For this review, take the finished solid that the model builds, in its own axes (mm). A direction names the side the tool comes from. Round coordinates to 2 decimals unless told otherwise and drop trailing zeros. Loops run counter-clockwise (first coordinate to the right, second up) from the corner with the lowest first, then second, coordinate; pieces in that order, holes last.
```python
from build123d import *
from OCP.BRepFilletAPI import BRepFilletAPI_MakeChamfer

# Parameters (mm, degrees)
ESQUISSE2_W             = 25
ESQUISSE2_H             = 36
BOSS_EXTRU_1_DEPTH      = 1.5
ESQUISSE3_W             = 3.350614404
ESQUISSE3_H             = 24
ESQUISSE3_W_2           = 3.329385596
BOSS_EXTRU_2_DEPTH      = 1.5
BOSS_EXTRU_3_DEPTH      = 8.58
BOSS_EXTRU_3_DEPTH_BACK = 3
BOSS_EXTRU_4_START      = 2.5
ESQUISSE5_W             = 18.32
ESQUISSE5_H             = 3
BOSS_EXTRU_4_DEPTH      = 6.08
ESQUISSE6_W             = 16.5
ESQUISSE6_H             = 1.5
BOSS_EXTRU_5_DEPTH      = 8
ESQUISSE7_W             = 25
ESQUISSE7_H             = 18
ENL_V_MAT_EXTRU_1_DEPTH = 5
CHANFREIN1_SIZE         = 10
CHANFREIN1_SIZE_2       = 5
CHANFREIN3_SIZE         = 3
CONG_1_R                = 3
CONG_2_R                = 3
D_GAGEMENT_M31_D        = 3.4


# Some blends are built 0.0001 mm under size
with BuildPart() as part:
    # Esquisse2 → Boss.-Extru.1 (new body)
    with BuildSketch(Plane.XY):
        with Locations((0, -137)):
            Rectangle(ESQUISSE2_W, ESQUISSE2_H)
    extrude(amount=BOSS_EXTRU_1_DEPTH)

    # Esquisse3 → Boss.-Extru.2 (add)
    with BuildSketch(Plane.XY.offset(1.5)):
        with Locations((10.824692798, -131)):
            Rectangle(ESQUISSE3_W, ESQUISSE3_H)
        Polygon((-12.5, -143), (-12.5, -155), (12.5, -155), (12.5, -143), (9.149385596, -143), (-9.170614404, -143), align=None)
        with Locations((-10.835307202, -131)):
            Rectangle(ESQUISSE3_W_2, ESQUISSE3_H)
    extrude(amount=BOSS_EXTRU_2_DEPTH)

    # Esquisse4 → Boss.-Extru.3 (add, two sides: drawn at the far end of the back side and taken through both)
    with BuildSketch(Plane.XY.offset(3).offset(-BOSS_EXTRU_3_DEPTH_BACK)):
        Polygon((-12.5, -119), (-15.5, -119), (-12.5, -137), (-12.5, -155), (12.5, -155), (12.5, -137), (15.5, -119), (12.5, -119), (10.747346399, -119), (10.747346399, -146), (-10.752653601, -146), (-10.752653601, -119), align=None)
    extrude(amount=BOSS_EXTRU_3_DEPTH + BOSS_EXTRU_3_DEPTH_BACK)

    # Esquisse5 → Boss.-Extru.4 (add)
    with BuildSketch(Plane.XY.offset(3).offset(BOSS_EXTRU_4_START)):
        Polygon((-10.752653601, -140), (-10.752653601, -146), (10.747346399, -146), (10.747346399, -140), (9.149385596, -140), (9.149385596, -143), (-9.170614404, -143), (-9.170614404, -140), align=None)
        with Locations((-0.010614404, -141.5)):
            Rectangle(ESQUISSE5_W, ESQUISSE5_H)
    extrude(amount=BOSS_EXTRU_4_DEPTH)

    # Esquisse6 → Boss.-Extru.5 (add)
    with BuildSketch(Plane(origin=(0, -119, 0), x_dir=(1, 0, 0), z_dir=(0, 1, 0))):
        Polygon((8.247346399, -11.58), (10.747346399, -11.58), (10.747346399, -5.5), (8.247346399, -5.5), (8.247346399, -10.08), align=None)
        with Locations((-0.002653601, -10.83)):
            Rectangle(ESQUISSE6_W, ESQUISSE6_H)
        Polygon((-10.752653601, -11.58), (-8.252653601, -11.58), (-8.252653601, -10.08), (-8.252653601, -5.5), (-10.752653601, -5.5), align=None)
    extrude(amount=-BOSS_EXTRU_5_DEPTH)

    # Esquisse7 → Enlèv. mat.-Extru.1 (cut)
    with BuildSketch(Plane.XY.offset(11.58)):
        with Locations((0, -146)):
            Rectangle(ESQUISSE7_W, ESQUISSE7_H)
    extrude(amount=-ENL_V_MAT_EXTRU_1_DEPTH, mode=Mode.SUBTRACT)

    # Chanfrein1
    chanfrein1_edges_1 = [part.edges().sort_by_distance(p)[0] for p in [
        (11.6236732, -137, 11.58),
    ]]
    chanfrein1_side_1 = [part.faces().sort_by_distance(p)[0] for p in [
        (11.6236732, -136.9, 11.58),
    ]]
    chanfrein1_edges_2 = [part.edges().sort_by_distance(p)[0] for p in [
        (-11.6263268, -137, 11.58),
    ]]
    chanfrein1_side_2 = [part.faces().sort_by_distance(p)[0] for p in [
        (-11.6263268, -136.9, 11.58),
    ]]
    chanfrein1 = BRepFilletAPI_MakeChamfer(part.part.solid().wrapped)
    for e in chanfrein1_edges_1:
        chanfrein1.Add(CHANFREIN1_SIZE - 0.0001, CHANFREIN1_SIZE_2 - 0.0001, e.wrapped, chanfrein1_side_1[0].wrapped)
    for e in chanfrein1_edges_2:
        chanfrein1.Add(CHANFREIN1_SIZE - 0.0001, CHANFREIN1_SIZE_2 - 0.0001, e.wrapped, chanfrein1_side_2[0].wrapped)
    add(Compound.cast(chanfrein1.Shape()), mode=Mode.REPLACE)  # a hair under: the kernel refuses the full size

    # Chanfrein3
    # the kernel refuses this chamfer: 3 mm, written as the material it adds along each edge
    with BuildSketch(Plane(origin=(-10.752653601, -127, 5.5), x_dir=(0.9996219169112968, 0.027495876610586775, 0), z_dir=(0, 0, 1))) as chanfrein3_piece_1_section:
        Polygon((CHANFREIN3_SIZE * 0.999621916911, -CHANFREIN3_SIZE * 0.0274958766106), (-CHANFREIN3_SIZE * 0.0274958766106, -CHANFREIN3_SIZE * 0.999621916911), (0, 0), align=None)
    chanfrein3_piece_1 = extrude(amount=6.08, mode=Mode.PRIVATE)
    chanfrein3_piece_1 = split(chanfrein3_piece_1, bisect_by=Plane(origin=(-8.784858651, -128.928894575, 10.615612357), z_dir=(0, 0.4472100177446834, -0.8944289798686087)), keep=Keep.TOP, mode=Mode.PRIVATE)
    chanfrein3_piece_1 = split(chanfrein3_piece_1, bisect_by=Plane(origin=(-8.252653601, -127.516102525, 7.79), z_dir=(-1, 0, 0)), keep=Keep.TOP, mode=Mode.PRIVATE)
    add(chanfrein3_piece_1)
    with BuildSketch(Plane(origin=(-10.752653601, -127, -2.215048964), x_dir=(0.9996219169112968, 0.027495876610586775, 0), z_dir=(0, 0, 1))) as chanfrein3_piece_2_section:
        Polygon((CHANFREIN3_SIZE * 0.999621916911, -CHANFREIN3_SIZE * 0.0274958766106), (-CHANFREIN3_SIZE * 0.0274958766106, -CHANFREIN3_SIZE * 0.999621916911), (0, 0), align=None)
    chanfrein3_piece_2 = extrude(amount=13.795048964, mode=Mode.PRIVATE)
    chanfrein3_piece_2 = split(chanfrein3_piece_2, bisect_by=Plane(origin=(-8.083536067, -127.445596899, 11.357253778), z_dir=(0, 0.4472100177446834, -0.8944289798686087)), keep=Keep.TOP, mode=Mode.PRIVATE)
    chanfrein3_piece_2 = split(chanfrein3_piece_2, bisect_by=Plane(origin=(-8.083536067, -127.161764932, 10.08), z_dir=(0, 0, 1)), keep=Keep.TOP, mode=Mode.PRIVATE)
    add(chanfrein3_piece_2)
    with BuildSketch(Plane(origin=(10.747346399, -127, 11.58), x_dir=(0.027495876610588044, -0.9996219169112968, 0), z_dir=(0, 0, -1))) as chanfrein3_piece_3_section:
        Polygon((CHANFREIN3_SIZE * 0.999621916911, CHANFREIN3_SIZE * 0.0274958766106), (-CHANFREIN3_SIZE * 0.0274958766106, CHANFREIN3_SIZE * 0.999621916911), (0, 0), align=None)
    chanfrein3_piece_3 = extrude(amount=6.08, mode=Mode.PRIVATE)
    chanfrein3_piece_3 = split(chanfrein3_piece_3, bisect_by=Plane(origin=(9.990097255, -128.087123339, 11.036493766), z_dir=(0, 0.4472100177446834, -0.8944289798686087)), keep=Keep.TOP, mode=Mode.PRIVATE)
    chanfrein3_piece_3 = split(chanfrein3_piece_3, bisect_by=Plane(origin=(8.247346399, -127.874570821, 10.61138448), z_dir=(1, 0, 0)), keep=Keep.TOP, mode=Mode.PRIVATE)
    add(chanfrein3_piece_3)
    with BuildSketch(Plane(origin=(10.747346399, -127, 11.58), x_dir=(0.027495876610588044, -0.9996219169112968, 0), z_dir=(0, 0, -1))) as chanfrein3_piece_4_section:
        Polygon((CHANFREIN3_SIZE * 0.999621916911, CHANFREIN3_SIZE * 0.0274958766106), (-CHANFREIN3_SIZE * 0.0274958766106, CHANFREIN3_SIZE * 0.999621916911), (0, 0), align=None)
    chanfrein3_piece_4 = extrude(amount=13.795048964, mode=Mode.PRIVATE)
    chanfrein3_piece_4 = split(chanfrein3_piece_4, bisect_by=Plane(origin=(8.078228865, -127.445596899, 11.357253778), z_dir=(0, 0.4472100177446834, -0.8944289798686087)), keep=Keep.TOP, mode=Mode.PRIVATE)
    chanfrein3_piece_4 = split(chanfrein3_piece_4, bisect_by=Plane(origin=(8.078228865, -127.161764932, 10.08), z_dir=(0, 0, 1)), keep=Keep.TOP, mode=Mode.PRIVATE)
    add(chanfrein3_piece_4)

    # Congé1
    cong_1_edges = [part.edges().sort_by_distance(p)[0] for p in [
        (-15.5, -119, 5.79),
        (15.5, -119, 5.79),
    ]]
    fillet(cong_1_edges, radius=CONG_1_R)

    # Congé2
    cong_2_edges = [part.edges().sort_by_distance(p)[0] for p in [
        (12.5, -155, 3.29),
        (-12.5, -155, 3.29),
    ]]
    fillet(cong_2_edges, radius=CONG_2_R)

    # Dégagement M31 (through all)
    with Locations(Plane.XY.offset(6.58)):
        with Locations((7.5, -149), (-7.5, -149)):
            Hole(D_GAGEMENT_M31_D / 2)


solid = part.part
```
(1) Insertion check: pin 1 Ø5.5 at (x, y) = (-2, -136) entering from +Z; pin 2 Ø3.5 at (y, z) = (-146.5, 3) entering from +X; pin 3 Ø3 at (x, y) = (7.5, -149) entering from -Z; pin 4 Ø1.6 at (x, z) = (0, 2.5) entering from +Y. Each pin has a flat end and moves straight along its axis. Give the tip position at first contact, or say it passes through.
(2) For L1, parallel to X at y = -149, z = 2.5; L2, parallel to Y at x = 7.5, z = 1.75; L3, parallel to X at y = -139, z = 2.5, list the stretches that pass through material, from the lowest coordinate up.
(3) Add section A-A (x = -0.5). Give the boundary of the cut face in (y, z).
(4) The part is to be moulded in two halves that separate along Z. For faces 1 (the cylindrical face through (7.87, -150.66, 3.24)), 2 (the flat face through (11.63, -130.82, 9.67)), 3 (the flat face through (-9, -124, 5.5)), say which applies: pulls with the +Z half, pulls with the -Z half, needs draft (parallel to the pull), parting line crosses it, or undercut.
(5) Add section C-C (y = -149). Give the boundary of the cut face in (x, z).
(6) For faces 4 (the flat face through (12.5, -145, 3)), 5 (the flat face through (0, -140, 6)), 6 (the flat face through (0, -131, 1.5)), list the 3-axis set-ups (+Z, -Z, +X, -X, +Y, -Y) from which the entire face can be reached by the end or side of a thin tool; tool diameter is ignored.
(7) Add section D-D (z = 4.75). Give the boundary of the cut face in (x, y), plus the area to 3 significant figures.
(8) Add section B-B (y = -123.5). Give the boundary of the cut face in (x, z), plus the area to 3 significant figures.
Outcome:
1. pin 1: stops at z = 1.5
1. pin 2: stops at x = 12.5
1. pin 3: passes through
1. pin 4: stops at y = -143
2. L1: x = -12.5 to -9.2, -5.8 to 5.8, 9.2 to 12.5
2. L2: y = -155 to -150.7, -147.3 to -143
2. L3: x = -12.5 to -9.17, 9.15 to 12.5
3. outline: (-155, 0) - (-119, 0) - (-119, 1.5) - (-143, 1.5) - (-143, 3) - (-146, 3) - (-146, 5.5) - (-140, 5.5) - (-140, 6.58) - (-155, 6.58) - close; (-127, 10.08) - (-119, 10.08) - (-119, 11.58) - (-127, 11.58) - close
4. face 1: needs draft
4. face 2: pulls with the +Z half
4. face 3: undercut
5. outline: (-12.5, 0) - (-9.2, 0) - (-9.2, 6.58) - (-12.5, 6.58) - close; (-5.8, 0) - (5.8, 0) - (5.8, 6.58) - (-5.8, 6.58) - close; (9.2, 0) - (12.5, 0) - (12.5, 6.58) - (9.2, 6.58) - close
6. face 4: +Z, -Z, +X, -Y
6. face 5: +Z
6. face 6: +Y
7. outline: (-14.92, -122.49) - (-12.5, -137) - (-12.5, -152) arc R3 ccw to (-9.5, -155) - (9.5, -155) arc R3 ccw to (12.5, -152) - (12.5, -137) - (14.92, -122.49) arc R3 ccw to (11.96, -119) - (10.75, -119) - (10.75, -146) - (-10.75, -146) - (-10.75, -119) - (-11.96, -119) arc R3 ccw to start; hole circle Ø3.4 at (-7.5, -149); hole circle Ø3.4 at (7.5, -149)
7. area: 346 mm2
8. outline: (-14.75, 0) - (14.75, 0) - (14.75, 11.58) - (-14.75, 11.58) - close; hole (-10.75, 3) - (-9.17, 3) - (-9.17, 1.5) - (9.15, 1.5) - (9.15, 3) - (10.75, 3) - (10.75, 5.5) - (8.25, 5.5) - (8.25, 10.08) - (-8.25, 10.08) - (-8.25, 5.5) - (-10.75, 5.5) - close
8. area: 185 mm2
